Part model, mm, in its own coordinate system. Coordinates: 2 decimals unless noted, no trailing zeros. Order: outer loops, then holes, each group sorted by start corner. A loop starts at its lowest first (then second) coordinate and runs counter-clockwise, first axis right, second up. Notation, with made-up numbers: (26.5, -27.5) - (52.5, -27.5) arc R24 cw to (52.5, 3.5) - close; hole circle Ø1 at (78, 63.5). An arc over 180 degrees is marked (long way). Use a Markdown table: item, result. Add a question column.
1) Saw through at B-B on x = 55. List the corners of the cut face in (y, z).
2) Wall check: L1, parallel to Y at x = 25, z = 7.75; L2, parallel to X at y = 82, z = 5.25; L3, parallel to X at y = 70, z = 6 (3 decimals). Give the ranges that are in metal, low to high. Write a range as [from, to].
3) Saw through at A-A on y = 8. List the corners of the cut face in (x, z), then the cut area to 4 significant figures.
4) Two-plate mould, pull along Y, no slides. Class faces 1 (the face through (59.048, 21.391, 4.698)), 2 (the face through (0, 44, 5)), 3 (the face through (39, 0, 5)): +Y half, -Y half, draft (parallel to the pull), parting line (faces both ways), or undercut.
```python
from build123d import *

# Parameters (mm, degrees)
SKETCH1_W             = 80
SKETCH1_H             = 90
SKETCH1_R             = 1.65
BOSS_EXTRUDE1_DEPTH   = 9.53
M4X0_7_TAPPED_HOLE1_D = 3.3
M4X0_7_TAPPED_HOLE2_D = 3.3


with BuildPart() as part:
    # Sketch1 → Boss-Extrude1 (new body)
    # profile 1 of 5: a face of its own
    with BuildSketch(Plane.XY):
        with Locations((40, 45)):
            Rectangle(SKETCH1_W, SKETCH1_H)
        with Locations((25, 82)):
            Circle(SKETCH1_R, mode=Mode.SUBTRACT)
        with Locations((55, 82)):
            Circle(SKETCH1_R, mode=Mode.SUBTRACT)
        with Locations((25, 8)):
            Circle(SKETCH1_R, mode=Mode.SUBTRACT)
        with Locations((55, 8)):
            Circle(SKETCH1_R, mode=Mode.SUBTRACT)
    # profile 2 of 5: a face of its own
    with BuildSketch(Plane.XY):
        with Locations((25, 8)):
            Circle(SKETCH1_R)
    # profile 3 of 5: a face of its own
    with BuildSketch(Plane.XY):
        with Locations((55, 8)):
            Circle(SKETCH1_R)
    # profile 4 of 5: a face of its own
    with BuildSketch(Plane.XY):
        with Locations((55, 82)):
            Circle(SKETCH1_R)
    # profile 5 of 5: a face of its own
    with BuildSketch(Plane.XY):
        with Locations((25, 82)):
            Circle(SKETCH1_R)
    extrude(amount=BOSS_EXTRUDE1_DEPTH)

    # M4x0.7 Tapped Hole1 (through all)
    with Locations(Plane(origin=(20.065, 70, 9.53), x_dir=(1, 0, 0), z_dir=(0, 0, 1))):
        with Locations((0, 0), (39.87, 0), (39.87, -50), (0, -50)):
            Hole(M4X0_7_TAPPED_HOLE1_D / 2)

    # M4x0.7 Tapped Hole2 (through all)
    with Locations(Plane(origin=(55, 8, 0), x_dir=(-1, 0, 0), z_dir=(0, 0, -1))):
        with Locations((0, 0), (30, 0), (30, 74), (0, 74)):
            Hole(M4X0_7_TAPPED_HOLE2_D / 2)


solid = part.part
```
Results are:
| question | item | result |
|---|---|---|
| 1 | outline | (0, 0) - (6.35, 0) - (6.35, 9.53) - (0, 9.53) - close; (9.65, 0) - (80.35, 0) - (80.35, 9.53) - (9.65, 9.53) - close; (83.65, 0) - (90, 0) - (90, 9.53) - (83.65, 9.53) - close |
| 2 | L1 | [0, 6.35], [9.65, 80.35], [83.65, 90] |
| 2 | L2 | [0, 23.35], [26.65, 53.35], [56.65, 80] |
| 2 | L3 | [0, 18.415], [21.715, 58.285], [61.585, 80] |
| 3 | outline | (0, 0) - (23.35, 0) - (23.35, 9.53) - (0, 9.53) - close; (26.65, 0) - (53.35, 0) - (53.35, 9.53) - (26.65, 9.53) - close; (56.65, 0) - (80, 0) - (80, 9.53) - (56.65, 9.53) - close |
| 3 | area | 699.5 mm2 |
| 4 | face 1 | undercut |
| 4 | face 2 | draft |
| 4 | face 3 | -Y half |
